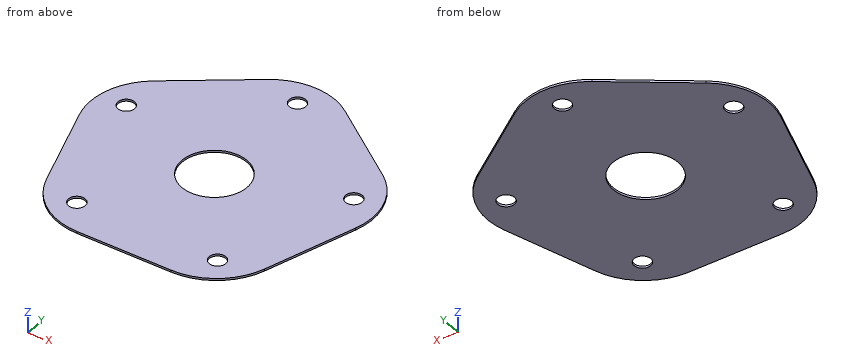
Solid Edge part; units mm, degrees
sketch "Sketch1" plane through (0, 0, 0) normal (0, 0, -1) x (-1, 0, 0)
  line L0 (-9.1636, 31.6216) -> (-27.2423, 18.4866)
  arc A0 (-27.2423, 18.4866) -> (-32.9056, 1.0566) centre (-18.0788, 5.8742) ccw
  line L1 (-32.9056, 1.0566) -> (-26.0002, -20.1962)
  arc A1 (-26.0002, -20.1962) -> (-11.1732, -30.9686) centre (-11.1732, -15.3786) ccw
  line L2 (-11.1732, -30.9686) -> (11.1732, -30.9686)
  arc A2 (26.0002, -20.1962) -> (11.1732, -30.9686) centre (11.1732, -15.3786) cw
  line L3 (26.0002, -20.1962) -> (32.9056, 1.0565)
  arc A3 (32.9056, 1.0565) -> (27.2422, 18.4867) centre (18.0786, 5.8741) ccw
  line L4 (27.2422, 18.4867) -> (9.1636, 31.6216)
  arc A4 (9.1636, 31.6216) -> (-9.1636, 31.6216) centre (0, 19.009) ccw
extrude "Protrusion1" add sketch "Sketch1" along normal blind 0.5
hole "Furat_1" at (27.1051, 8.807, -0.5) direction (0, 0, 1) diameter 4 end through all
pattern_circular "MintaElőfordulás_1" count 5 over 360 about axis through (0, 0, -0.5) along (0, 0, 1) of "Furat_1"
sketch "Sketch2" plane through (0, 1.8152, -0.5) normal (0, 0, -1) x (-0.309017, 0.9510565, 0)
  circle A0 centre (-1.7263, -0.5609) radius 7.8
extrude "Kivágás_1" cut sketch "Sketch2" against normal blind 32.365
properties material "Szilikon"
Check sheet for the modelled part. Datum: model origin and axes. Units: mm. Round coordinates to 2 decimals unless told otherwise and drop trailing zeros. Loops run counter-clockwise (first coordinate to the right, second up) from the corner with the lowest first, then second, coordinate; pieces in that order, holes last.
1. Scan lines: probe 1 along Y at (x, z) = (17, -0.25); probe 2 along X at (y, z) = (2, -0.25); probe 3 along Y at (x, z) = (-2.5, -0.15). Record each from-to range of solid material in increasing order.
2. Sectioned sample at D-D on x = -13.5. Record the boundary of the cut face in (y, z), and give its area (3 significant figures).
3. Sectioned sample at B-B on y = -7. Record the boundary of the cut face in (x, z), and give its area (3 significant figures).
4. Gauge pin test, flat end, axial feed: pin 1 Ø3 at (x, y) = (0, 28.5) entering from -Z. Record the tip position at first contact, or that the pin passes through.
5. Sectioned sample at A-A on x = 3. Record the boundary of the cut face in (y, z), and give its area (3 significant figures).
Recorded:
1. probe 1: y = -29.84 to -25.04, -21.07 to 25.93
1. probe 2: x = -33.18 to -7.54, 7.54 to 33.18
1. probe 3: y = -30.97 to -7.39, 7.39 to 34.4
2. outline: (-30.79, -0.5) - (28.47, -0.5) - (28.47, 0) - (-30.79, 0) - close
2. area: 29.6 mm2
3. outline: (-30.29, -0.5) - (-3.44, -0.5) - (-3.44, 0) - (-30.29, 0) - close; (3.44, -0.5) - (30.29, -0.5) - (30.29, 0) - (3.44, 0) - close
3. area: 26.8 mm2
4. pin 1: passes through
5. outline: (-30.97, -0.5) - (-7.2, -0.5) - (-7.2, 0) - (-30.97, 0) - close; (7.2, -0.5) - (34.31, -0.5) - (34.31, 0) - (7.2, 0) - close
5. area: 25.4 mm2
